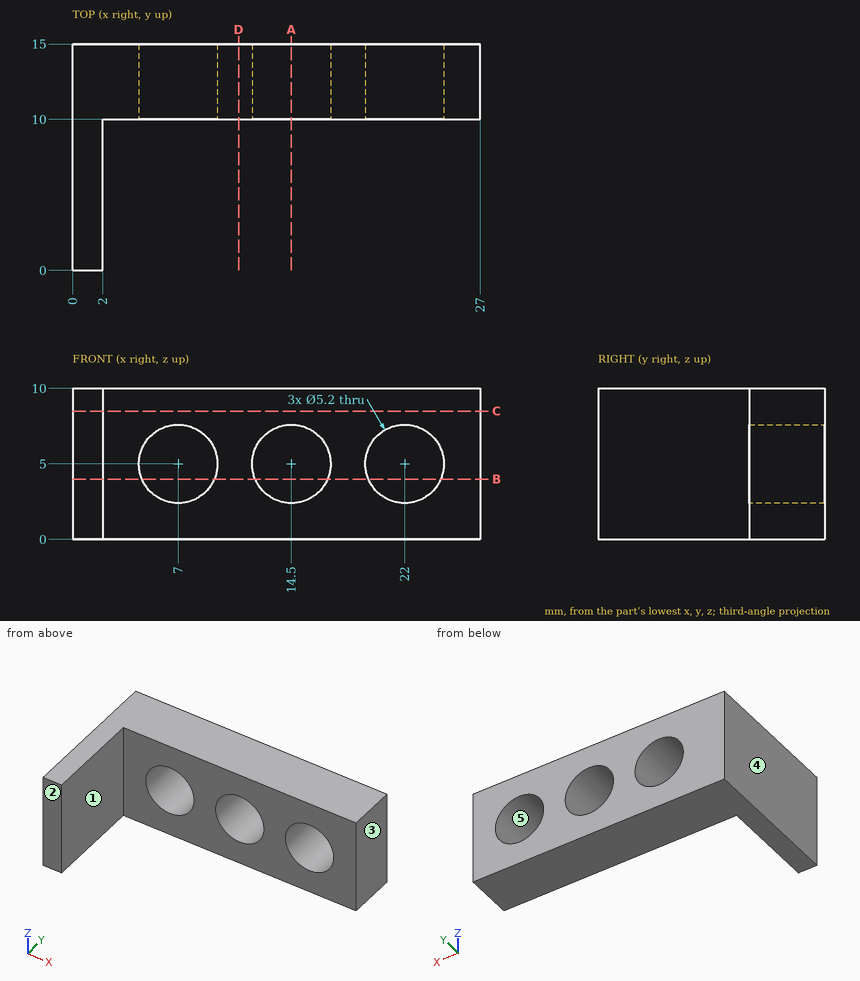
Verification items for this drawing (mm, ordinates from the low corner). A direction names the side the tool comes from. Coordinates: 2 decimals unless noted, no trailing zeros. Order: outer loops, then holes, each group sorted by start corner. A loop starts at its lowest first (then second) coordinate and runs counter-clockwise, first axis right, second up. Notation, with made-up numbers: (-9, 78.25) - (17, 78.25) arc R23 ccw to (17, 103.25) - close; hole circle Ø11 at (48, 29). An arc over 180 degrees is marked (long way). Use one line per item in the form item = value.
1. Draft check along X on the marked faces 3, 4 and 5. Enter one of: pulls with the +X half, pulls with the -X half, needs draft (parallel to the pull), parting line crosses it, or undercut.
Here are the results:
face_3 = pulls with the +X half
face_4 = pulls with the -X half
face_5 = undercut
2. Section check B-B (z = 4). Record the boundary of the cut face in (x, y), then the cut area to 3 significant figures.
Here are the results:
outline = (0, 0) - (2, 0) - (2, 10) - (4.6, 10) - (4.6, 15) - (0, 15) - close; (9.4, 10) - (12.1, 10) - (12.1, 15) - (9.4, 15) - close; (16.9, 10) - (19.6, 10) - (19.6, 15) - (16.9, 15) - close; (24.4, 10) - (27, 10) - (27, 15) - (24.4, 15) - close
area = 83.0 mm²
3. Section check D-D (x = 11). Record the boundary of the cut face in (y, z).
Here are the results:
outline = (10, 0) - (15, 0) - (15, 10) - (10, 10) - close
4. Gauge pin test, flat ends, axial feed: pin 1 (5 mm diameter, centred on y = 5, z = 5, fed in from +X); pin 2 (5 mm diameter, centred on x = 14, z = 6.5, fed in from -Y). Record the tip position at first contact, or that the pin passes through.
Here are the results:
pin_1 = 2
pin_2 = 10
5. Section check A-A (x = 14.5). Record the boundary of the cut face in (y, z).
Here are the results:
outline = (10, 0) - (15, 0) - (15, 2.4) - (10, 2.4) - close; (10, 7.6) - (15, 7.6) - (15, 10) - (10, 10) - close
6. Access from +Z, -Z, +X, -X, +Y, -Y to the whole of each face (thin tool, end or side, straight path). Record for the marked faces 1 and 2.
Here are the results:
face_1 = +Z, -Z, +X, -Y
face_2 = +Z, -Z, +X, -X, -Y
7. Scan lines: line 1 (X direction, y = 11.5, z = 5); line 2 (Y direction, x = 17.5, z = 4.5); line 3 (X direction, y = 2.75, z = 5.75). Record each from-to range of solid material in increasing order.
Here are the results:
line_1 = 0 to 4.4, 9.6 to 11.9, 17.1 to 19.4, 24.6 to 27
line_2 = 10 to 15
line_3 = 0 to 2
8. Section check C-C (z = 8.5). Record the boundary of the cut face in (x, y), then the cut area to 3 significant figures.
Here are the results:
outline = (0, 0) - (2, 0) - (2, 10) - (27, 10) - (27, 15) - (0, 15) - close
area = 155 mm²
